Could you check a few things on this model? Use its own coordinates, in mm. Face numbers are marked on the shaded views. A direction names the side the tool comes from. Give positions to 0.01 mm unless a question says otherwise; leave off trailing zeros. Loops run counter-clockwise (first coordinate to the right, second up) from the corner with the lowest first, then second, coordinate; pieces in that order, holes last. Notation, with made-up numbers: M -9.75,1 L 23.25,1 A21 cw 23.25,24 Z; hole C 43.25,-21 d4. An arc over 180 degrees is marked long. Use a Markdown table: item, result. Add a question column.
1) We'd pull the mould along Y, two halves only. Please class the marked faces 1, 2 and 3: +Y half, -Y half, draft (parallel to the pull), parting line (faces both ways), or undercut.
2) Suppose I cut it at A-A on z = 18.75. List the corners of the cut face in (x, y) for me, and give its area (3 significant figures).
3) Suppose I cut it at C-C on y = 33. List the corners of the cut face in (x, z) for me, and give its area (3 significant figures).
4) Will these pins go through, and if not, where does the flat tip stop? pin 1 Ø4 at (x, z) = (-14, 4.5) entering from +Y; pin 2 Ø2.5 at (x, z) = (-12, 5) entering from -Y; pin 3 Ø10 at (x, z) = (-2.5, 8.5) entering from +Y; pin 4 Ø5 at (x, y) = (-57, 19) entering from -Z.
5) Which directions (+Z, -Z, +X, -X, +Y, -Y) give clear straight access to the entire face, cutting with the end or side of a thin tool? Please do the marked faces 4, 5 and 6.
6) Suppose I cut it at B-B on y = 11.5. List the corners of the cut face in (x, z) for me.
7) If I drill on line 1 along Y through (x, z) = (-26, 5.5); line 2 along X through (y, z) = (26.5, 5.5); line 3 along Y through (x, z) = (0.5, 14.5), over which ranges is the centre line in solid material (lowest first)? Write a range as [from, to].
```python
from build123d import *

# Parameters (mm, degrees)
CROQUIS1_R                 = 1.5
SALIENTE_EXTRUIR1_DEPTH    = 2.4
CROQUIS3_W                 = 25.05
CROQUIS3_H                 = 24.65
CROQUIS3_W_2               = 22.65
CROQUIS3_H_2               = 22.25
SALIENTE_EXTRUIR2_DEPTH    = 10
CROQUIS4_W                 = 25.05
CROQUIS4_H                 = 24.65
CROQUIS4_W_2               = 17.05
CROQUIS4_H_2               = 16.65
SALIENTE_EXTRUIR3_DEPTH    = 1.2
CROQUIS5_W                 = 4
CROQUIS5_H                 = 2.5
CROQUIS5_W_2               = 15.15
CROQUIS5_H_2               = 4
CROQUIS5_H_3               = 1
CORTAR_EXTRUIR1_DEPTH      = 11.2
CROQUIS8_W                 = 15
CROQUIS8_H                 = 15
SALIENTE_EXTRUIR5_DEPTH    = 15
CROQUIS10_R                = 5
CORTAR_EXTRUIR2_DEPTH      = 5
CORTAR_EXTRUIR3_START      = -10
CROQUIS10_2_R              = 5
CORTAR_EXTRUIR3_DEPTH      = 5
CROQUIS11_R                = 3.5
CORTAR_EXTRUIR4_DEPTH      = 5
CORTAR_EXTRUIR5_DEPTH      = 2.4
CORTAR_EXTRUIR6_DEPTH      = 10
CORTAR_EXTRUIR6_DEPTH_BACK = 2.4
CROQUIS13_W                = 10
CROQUIS13_H                = 4.5
REDONDEO1_R                = 5
CORTAR_EXTRUIR7_REACH      = 92.864
CROQUIS14_W                = 37
CROQUIS14_H                = 25
CROQUIS14_W_2              = 3
CROQUIS14_H_2              = 2
SALIENTE_EXTRUIR6_DEPTH    = 3.6
SALIENTE_EXTRUIR7_DEPTH    = 1.2
SALIENTE_EXTRUIR8_DEPTH    = 5
CORTAR_EXTRUIR8_DEPTH      = 5.000001
CROQUIS25_R                = 2.5
SALIENTE_EXTRUIR9_DEPTH    = 2


with BuildPart() as part:
    # Croquis1 → Saliente-Extruir1 (new body)
    with BuildSketch(Plane.XY):
        with BuildLine():
            Line((-65.940699516, 48.688511327), (-65.940699516, 17.688511327))
            ThreePointArc((-65.940699516, 17.688511327), (-64.76912664, 14.860084202), (-61.940699516, 13.688511327))
            ThreePointArc((-61.940699516, 13.688511327), (-28.440699516, 5.688511327), (5.059300484, 13.688511327))
            ThreePointArc((5.059300484, 13.688511327), (9.059300484, 17.688511327), (5.059300484, 21.688511327))
            ThreePointArc((5.059300484, 21.688511327), (-6.440699516, 33.188511327), (5.059300484, 44.688511327))
            ThreePointArc((5.059300484, 44.688511327), (9.059300484, 48.688511327), (5.059300484, 52.688511327))
            ThreePointArc((5.059300484, 52.688511327), (-28.440699516, 60.688511327), (-61.940699516, 52.688511327))
            ThreePointArc((-61.940699516, 52.688511327), (-64.76912664, 51.516938452), (-65.940699516, 48.688511327))
        make_face()
        with Locations((-61.940699516, 48.688511327)):
            Circle(CROQUIS1_R, mode=Mode.SUBTRACT)
        with Locations((5.059300484, 48.688511327)):
            Circle(CROQUIS1_R, mode=Mode.SUBTRACT)
        with Locations((5.059300484, 17.688511327)):
            Circle(CROQUIS1_R, mode=Mode.SUBTRACT)
        with Locations((-61.940699516, 17.688511327)):
            Circle(CROQUIS1_R, mode=Mode.SUBTRACT)
    extrude(amount=SALIENTE_EXTRUIR1_DEPTH)

    # Croquis3 → Saliente-Extruir2 (add)
    with BuildSketch(Plane.XY.offset(2.4)):
        with Locations((-24.965699516, 42.160543548)):
            Rectangle(CROQUIS3_W, CROQUIS3_H)
        with Locations((-24.965699516, 42.160543548)):
            Rectangle(CROQUIS3_W_2, CROQUIS3_H_2, mode=Mode.SUBTRACT)
    extrude(amount=SALIENTE_EXTRUIR2_DEPTH)

    # Croquis4 → Saliente-Extruir3 (add)
    with BuildSketch(Plane.XY.offset(12.4)):
        with Locations((-24.965699516, 42.160543548)):
            Rectangle(CROQUIS4_W, CROQUIS4_H)
        with Locations((-24.965699516, 42.160543548)):
            Rectangle(CROQUIS4_W_2, CROQUIS4_H_2, mode=Mode.SUBTRACT)
    extrude(amount=SALIENTE_EXTRUIR3_DEPTH)

    # Croquis5 → Cortar-Extruir1 (cut)
    with BuildSketch(Plane.XY.offset(13.6)):
        with Locations((-35.490699516, 48.035543548)):
            Rectangle(CROQUIS5_W, CROQUIS5_H)
        with Locations((-24.015699516, 52.485543548)):
            Rectangle(CROQUIS5_W_2, CROQUIS5_H_2)
        with Locations((-14.440699516, 36.035543548)):
            Rectangle(CROQUIS5_W, CROQUIS5_H_3)
        with Locations((-14.440699516, 48.035543548)):
            Rectangle(CROQUIS5_W, CROQUIS5_H)
    extrude(amount=-CORTAR_EXTRUIR1_DEPTH, mode=Mode.SUBTRACT)

    # Croquis8 → Saliente-Extruir5 (add)
    with BuildSketch(Plane.XY.offset(2.4)):
        with Locations((-55.440699516, 33.188511327)):
            Rectangle(CROQUIS8_W, CROQUIS8_H)
    extrude(amount=SALIENTE_EXTRUIR5_DEPTH)

    # Croquis10 → Cortar-Extruir2 (cut)
    with BuildSketch(Plane.XZ.offset(-25.688511327)):
        with Locations(Location((-55.440699516, 9.9, 0), (0, 0, 270))):
            Circle(CROQUIS10_R)
    extrude(amount=-CORTAR_EXTRUIR2_DEPTH, mode=Mode.SUBTRACT)

    # Croquis10<2> → Cortar-Extruir3 (cut)
    with BuildSketch(Plane.XZ.offset(-25.688511327).offset(CORTAR_EXTRUIR3_START)):
        with Locations(Location((-55.440699516, 9.9, 0), (0, 0, 270))):
            Circle(CROQUIS10_2_R)
    extrude(amount=-CORTAR_EXTRUIR3_DEPTH, mode=Mode.SUBTRACT)

    # Croquis11 → Cortar-Extruir4 (cut)
    with BuildSketch(Plane.XZ.offset(-30.688511327)):
        with Locations(Location((-55.440699516, 9.9, 0), (0, 0, 270))):
            Circle(CROQUIS11_R)
    extrude(amount=-CORTAR_EXTRUIR4_DEPTH, mode=Mode.SUBTRACT)

    # Croquis12 → Cortar-Extruir5 (cut)
    with BuildSketch(Plane.XY.offset(2.4)):
        Polygon((-36.290699516, 53.285543548), (-13.640699516, 53.285543548), (-13.640699516, 49.285543548), (-8.640699516, 49.285543548), (-8.640699516, 46.785543548), (-13.640699516, 46.785543548), (-13.640699516, 31.035543548), (-36.290699516, 31.035543548), (-36.290699516, 46.785543548), (-41.290699516, 46.785543548), (-41.290699516, 49.285543548), (-36.290699516, 49.285543548), align=None)
    extrude(amount=-CORTAR_EXTRUIR5_DEPTH, mode=Mode.SUBTRACT)

    # Croquis13 → Cortar-Extruir6 (cut, two sides: drawn at the far end of the back side and taken through both)
    with BuildSketch(Plane.XY.offset(2.4).offset(-CORTAR_EXTRUIR6_DEPTH_BACK)):
        with Locations((-18.640699516, 55.535543548)):
            Rectangle(CROQUIS13_W, CROQUIS13_H)
    extrude(amount=CORTAR_EXTRUIR6_DEPTH + CORTAR_EXTRUIR6_DEPTH_BACK, mode=Mode.SUBTRACT)

    # Redondeo1
    redondeo1_edges = [part.edges().sort_by_distance(p)[0] for p in [
        (-62.940699516, 33.188511327, 17.4),
        (-47.940699516, 33.188511327, 17.4),
    ]]
    fillet(redondeo1_edges, radius=REDONDEO1_R)

    # Croquis14 → Cortar-Extruir7 (cut, up to next)
    with BuildSketch(Plane.XY.offset(2.4), mode=Mode.PRIVATE) as cortar_extruir7_sk1:
        with Locations((-26.440699516, 14.335543548)):
            Rectangle(CROQUIS14_W, CROQUIS14_H)
    cortar_extruir7_tool1 = extrude(cortar_extruir7_sk1.sketch, amount=-CORTAR_EXTRUIR7_REACH, mode=Mode.PRIVATE) & part.part
    # Croquis14 → Cortar-Extruir7 (cut, up to next)
    with BuildSketch(Plane.XY.offset(2.4), mode=Mode.PRIVATE) as cortar_extruir7_sk2:
        with Locations((-32.490699516, 28.835543548)):
            Rectangle(CROQUIS14_W_2, CROQUIS14_H_2)
    cortar_extruir7_tool2 = extrude(cortar_extruir7_sk2.sketch, amount=-CORTAR_EXTRUIR7_REACH, mode=Mode.PRIVATE) & part.part
    add(cortar_extruir7_tool1.solids().sort_by_distance((-26.4407, 14.335544, 2.4))[0], mode=Mode.SUBTRACT)
    add(cortar_extruir7_tool2.solids().sort_by_distance((-32.4907, 28.835544, 2.4))[0], mode=Mode.SUBTRACT)

    # Croquis15 → Saliente-Extruir6 (add)
    with BuildSketch(Plane.XY.offset(2.4)):
        with BuildLine():
            Line((-44.940699516, 7.547864372), (-44.940699516, 26.835543548))
            Line((-44.940699516, 26.835543548), (-33.990699516, 26.835543548))
            Line((-33.990699516, 26.835543548), (-33.990699516, 28.435543548))
            Line((-33.990699516, 28.435543548), (-46.540699516, 28.435543548))
            Line((-46.540699516, 28.435543548), (-46.540699516, 7.931832654))
            ThreePointArc((-46.540699516, 7.931832654), (-45.74176474, 7.73540971), (-44.940699516, 7.547864372))
        make_face()
        with BuildLine():
            Line((-7.940699516, 26.835543548), (-7.940699516, 8.578997552))
            ThreePointArc((-7.940699516, 8.578997552), (-7.139347833, 8.814456916), (-6.340699516, 9.058928786))
            Line((-6.340699516, 9.058928786), (-6.340699516, 28.435543548))
            Line((-6.340699516, 28.435543548), (-30.990699516, 28.435543548))
            Line((-30.990699516, 28.435543548), (-30.990699516, 26.835543548))
            Line((-30.990699516, 26.835543548), (-7.940699516, 26.835543548))
        make_face()
    extrude(amount=SALIENTE_EXTRUIR6_DEPTH)

    # Croquis16 → Saliente-Extruir7 (add)
    with BuildSketch(Plane.XY.offset(6)):
        with BuildLine():
            Line((-33.990699516, 28.435543548), (-46.540699516, 28.435543548))
            Line((-46.540699516, 28.435543548), (-46.540699516, 7.931832654))
            ThreePointArc((-46.540699516, 7.931832654), (-44.745749867, 7.50363869), (-42.940699516, 7.120249144))
            Line((-42.940699516, 7.120249144), (-42.940699516, 24.835543548))
            Line((-42.940699516, 24.835543548), (-33.990699516, 24.835543548))
            Line((-33.990699516, 24.835543548), (-33.990699516, 28.435543548))
        make_face()
        with BuildLine():
            Line((-30.990699516, 28.435543548), (-6.340699516, 28.435543548))
            Line((-6.340699516, 28.435543548), (-6.340699516, 9.058928786))
            ThreePointArc((-6.340699516, 9.058928786), (-8.134228504, 8.523600003), (-9.940699516, 8.033716728))
            Line((-9.940699516, 8.033716728), (-9.940699516, 24.835543548))
            Line((-9.940699516, 24.835543548), (-30.990699516, 24.835543548))
            Line((-30.990699516, 24.835543548), (-30.990699516, 28.435543548))
        make_face()
    extrude(amount=SALIENTE_EXTRUIR7_DEPTH)

    # Croquis20 → Saliente-Extruir8 (add)
    with BuildSketch(Plane.XZ.offset(-25.688511327)):
        with BuildLine():
            Line((-62.940699516, 2.4), (-62.940699516, 11.011952661))
            Line((-62.940699516, 11.011952661), (-60.839725603, 8.511570775))
            ThreePointArc((-60.839725603, 8.511570775), (-59.506404562, 5.553015225), (-58.73875169, 2.4))
            Line((-58.73875169, 2.4), (-62.940699516, 2.4))
        make_face()
        with BuildLine():
            Line((-47.940699516, 2.4), (-47.940699516, 11.849634175))
            Line((-47.940699516, 11.849634175), (-50.161985782, 8.702014116))
            ThreePointArc((-50.161985782, 8.702014116), (-51.018961055, 5.604072702), (-51.275019132, 2.4))
            Line((-51.275019132, 2.4), (-47.940699516, 2.4))
        make_face()
    saliente_extruir8 = extrude(amount=SALIENTE_EXTRUIR8_DEPTH)

    # Simetría1: Saliente-Extruir8 across plane
    add(saliente_extruir8.mirror(Plane(origin=(0, 33.188511327, 0), x_dir=(0, 0, 1), z_dir=(0, -1, 0))))

    # Croquis22 → Cortar-Extruir8 (cut)
    with BuildSketch(Plane(origin=(0, 45.688511327, 0), x_dir=(1, 0, 0), z_dir=(0, 1, 0))):
        Polygon((-47.940699516, -11.849634175), (-49.670456383, -9.398523981), (-47.940699516, -8.17782863), align=None)
    extrude(amount=-CORTAR_EXTRUIR8_DEPTH, mode=Mode.SUBTRACT)

    # Croquis25 → Saliente-Extruir9 (add)
    with BuildSketch(Plane(origin=(0, 21.941734011, 0), x_dir=(1, 0, 0), z_dir=(0, 1, 0))):
        with BuildLine():
            Line((-6.340699516, -22.4), (-6.340699516, -2.4))
            Line((-6.340699516, -2.4), (2.659300484, -2.4))
            Line((2.659300484, -2.4), (2.659300484, -22.4))
            ThreePointArc((2.659300484, -22.4), (-1.840699516, -26.9), (-6.340699516, -22.4))
        make_face()
        with Locations(Location((-1.840699516, -22.4, 0), (0, 0, 270))):
            Circle(CROQUIS25_R, mode=Mode.SUBTRACT)
    saliente_extruir9 = extrude(amount=-SALIENTE_EXTRUIR9_DEPTH)

    # Simetría2: Saliente-Extruir9 across plane
    add(saliente_extruir9.mirror(Plane(origin=(0, 33.188511327, 0), x_dir=(0, 0, 1), z_dir=(0, -1, 0))))


solid = part.part
```
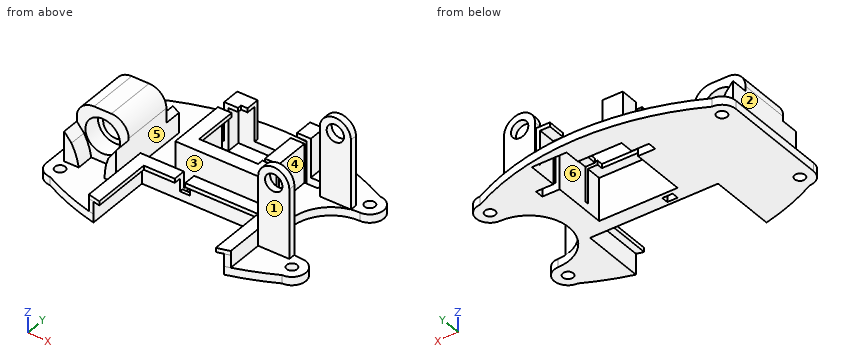
Answer block:
| question | item | result |
|---|---|---|
| 1 | face 1 | -Y half |
| 1 | face 2 | draft |
| 1 | face 3 | undercut |
| 2 | outline | M -6.34,19.94 L 2.66,19.94 L 2.66,21.94 L -6.34,21.94 Z; M -6.34,44.44 L 2.66,44.44 L 2.66,46.44 L -6.34,46.44 Z |
| 2 | area | 36.0 mm^2 |
| 3 | outline | M -65.94,0 L -36.29,0 L -36.29,12.4 L -13.64,12.4 L -13.64,0 L -6.44,0 L -6.44,2.4 L -12.44,2.4 L -12.44,13.6 L -37.49,13.6 L -37.49,2.4 L -47.94,2.4 L -47.94,12.4 A5 ccw -52.94,17.4 L -57.94,17.4 A5 ccw -62.94,12.4 L -62.94,2.4 L -65.94,2.4 Z; hole C -55.44,9.9 d7 |
| 3 | area | 318 mm^2 |
| 4 | pin 1 | stops at y = 54.49 |
| 4 | pin 2 | stops at y = 24.84 |
| 4 | pin 3 | stops at y = 46.44 |
| 4 | pin 4 | stops at z = 0 |
| 5 | face 4 | +Z, +Y |
| 5 | face 5 | +Z, +Y, -Y |
| 5 | face 6 | -Z |
| 6 | outline | M -57.22,0 L -44.94,0 L -44.94,6 L -42.94,6 L -42.94,7.2 L -46.54,7.2 L -46.54,2.4 L -57.22,2.4 Z; M -9.94,6 L -7.94,6 L -7.94,0 L 0.33,0 L 0.33,2.4 L -6.34,2.4 L -6.34,7.2 L -9.94,7.2 Z |
| 7 | line 1 | y = [26.84, 28.44], [29.84, 31.04] |
| 7 | line 2 | x = [-62.94, -57.82], [-53.07, -47.94], [-46.54, -44.94], [-7.94, -6.34] |
| 7 | line 3 | y = [19.94, 21.94], [44.44, 46.44] |
